```python
from build123d import *

# Parameters (mm, degrees)
BASE_FLANGE1_DEPTH = 156
SKETCH6_R          = 13
CUT_EXTRUDE1_DEPTH = 312.184832535
SKETCH7_R          = 21.05
SKETCH7_R_2        = 2.5
CUT_EXTRUDE2_DEPTH = 10
SKETCH9_R          = 19.05
SKETCH9_R_2        = 2.5
CUT_EXTRUDE3_DEPTH = 10
SKETCH10_R         = 13
CUT_EXTRUDE4_DEPTH = 10
SKETCH12_R         = 13
CUT_EXTRUDE5_DEPTH = 10
SKETCH14_R         = 3
CUT_EXTRUDE6_DEPTH = 10
SKETCH15_R         = 3
CUT_EXTRUDE7_DEPTH = 10
CUT_EXTRUDE8_DEPTH = 312.184832535
FILLET1_R          = 50
FILLET2_R          = 40
SKETCH16_R         = 3
CUT_EXTRUDE9_DEPTH = 10


# Sheet-metal steps are written as plain solids
with BuildPart() as part:
    # Sketch1 → Base-Flange1 (new body)
    with BuildSketch(Plane.XY):
        with BuildLine():
            Line((-77.380352645, 230), (-77.380352645, 3))
            ThreePointArc((-77.380352645, 3), (-76.501672988, 0.878679656), (-74.380352645, 0))
            Line((-74.380352645, 0), (53.619647355, 0))
            ThreePointArc((53.619647355, 0), (55.740967699, 0.878679656), (56.619647355, 3))
            Line((56.619647355, 3), (56.619647355, 230))
            Line((56.619647355, 230), (59.619647355, 230))
            Line((59.619647355, 230), (59.619647355, 3))
            ThreePointArc((59.619647355, 3), (57.862288042, -1.242640687), (53.619647355, -3))
            Line((53.619647355, -3), (-74.380352645, -3))
            ThreePointArc((-74.380352645, -3), (-78.622993332, -1.242640687), (-80.380352645, 3))
            Line((-80.380352645, 3), (-80.380352645, 230))
            Line((-80.380352645, 230), (-77.380352645, 230))
        make_face()
    extrude(amount=BASE_FLANGE1_DEPTH)

    # Sketch6 → Cut-Extrude1 (cut, through all)
    with BuildSketch(Plane(origin=(59.619647355, 0, 0), x_dir=(0, 0, -1), z_dir=(1, 0, 0))):
        with Locations((-78, 197)):
            Circle(SKETCH6_R)
    extrude(amount=-CUT_EXTRUDE1_DEPTH, mode=Mode.SUBTRACT)

    # Sketch7 → Cut-Extrude2 (cut)
    with BuildSketch(Plane.ZY.offset(80.380352645)):
        with Locations(Location((114, 100, 0), (0, 0, 270))):
            Circle(SKETCH7_R)
        with Locations(Location((90.43, 123.57, 0), (0, 0, 270))):
            Circle(SKETCH7_R_2)
        with Locations(Location((137.57, 123.57, 0), (0, 0, 270))):
            Circle(SKETCH7_R_2)
        with Locations(Location((137.57, 76.43, 0), (0, 0, 270))):
            Circle(SKETCH7_R_2)
        with Locations(Location((90.43, 76.43, 0), (0, 0, 270))):
            Circle(SKETCH7_R_2)
    extrude(amount=-CUT_EXTRUDE2_DEPTH, mode=Mode.SUBTRACT)

    # Sketch9 → Cut-Extrude3 (cut)
    with BuildSketch(Plane(origin=(59.619647355, 0, 0), x_dir=(0, 0, -1), z_dir=(1, 0, 0))):
        with Locations((-114, 40)):
            Circle(SKETCH9_R)
        with Locations((-90.43, 63.57)):
            Circle(SKETCH9_R_2)
        with Locations((-137.57, 63.57)):
            Circle(SKETCH9_R_2)
        with Locations((-137.57, 16.43)):
            Circle(SKETCH9_R_2)
        with Locations((-90.43, 16.43)):
            Circle(SKETCH9_R_2)
    extrude(amount=-CUT_EXTRUDE3_DEPTH, mode=Mode.SUBTRACT)

    # Sketch10 → Cut-Extrude4 (cut)
    with BuildSketch(Plane(origin=(0, 0, 0), x_dir=(1, 0, 0), z_dir=(0, 1, 0))):
        with Locations(Location((-10.380352645, -78, 0), (0, 0, 270))):
            Circle(SKETCH10_R)
    extrude(amount=-CUT_EXTRUDE4_DEPTH, mode=Mode.SUBTRACT)

    # Sketch12 → Cut-Extrude5 (cut)
    with BuildSketch(Plane.XZ.offset(3)):
        with Locations(Location((5.789398738, 44.000000006, 0), (0, 0, 270))):
            Circle(SKETCH12_R)
    extrude(amount=-CUT_EXTRUDE5_DEPTH, mode=Mode.SUBTRACT)

    # Sketch14 → Cut-Extrude6 (cut)
    with BuildSketch(Plane(origin=(59.619647355, 0, 0), x_dir=(0, 0, -1), z_dir=(1, 0, 0))):
        with Locations((-52, 97)):
            Circle(SKETCH14_R)
        with BuildLine():
            ThreePointArc((-46.82612575, 119.41051149), (-68.263455967, 113.263455967), (-74.41051149, 91.82612575))
            ThreePointArc((-74.41051149, 91.82612575), (-70.812548133, 89.577868719), (-68.564291101, 93.175832076))
            ThreePointArc((-68.564291101, 93.175832076), (-64.02081528, 109.02081528), (-48.175832076, 113.564291101))
            ThreePointArc((-48.175832076, 113.564291101), (-44.577868719, 115.812548133), (-46.82612575, 119.41051149))
        make_face()
        with BuildLine():
            ThreePointArc((-41.427300446, 142.795393045), (-85.234018716, 130.234018716), (-97.795393045, 86.427300446))
            ThreePointArc((-97.795393045, 86.427300446), (-94.197429688, 84.179043415), (-91.949172656, 87.777006772))
            ThreePointArc((-91.949172656, 87.777006772), (-80.991378029, 125.991378029), (-42.777006772, 136.949172656))
            ThreePointArc((-42.777006772, 136.949172656), (-39.179043415, 139.197429688), (-41.427300446, 142.795393045))
        make_face()
    extrude(amount=-CUT_EXTRUDE6_DEPTH, mode=Mode.SUBTRACT)

    # Sketch15 → Cut-Extrude7 (cut)
    with BuildSketch(Plane(origin=(-77.380352645, 0, 0), x_dir=(0, 0, -1), z_dir=(1, 0, 0))):
        with Locations(Location((-43, 160, 0), (0, 0, 90))):
            Circle(SKETCH15_R)
        with BuildLine():
            ThreePointArc((-85.143312097, 179.651749171), (-86.695706867, 144.096063335), (-62.651749171, 117.856687903))
            ThreePointArc((-62.651749171, 117.856687903), (-59.329434049, 119.065911716), (-60.538657862, 122.388226838))
            ThreePointArc((-60.538657862, 122.388226838), (-81.997243763, 145.806164052), (-80.611773162, 177.538657862))
            ThreePointArc((-80.611773162, 177.538657862), (-81.820996975, 180.860972984), (-85.143312097, 179.651749171))
        make_face()
        with BuildLine():
            ThreePointArc((-63.845079102, 169.72022002), (-64.612930278, 152.133536704), (-52.72022002, 139.154920898))
            ThreePointArc((-52.72022002, 139.154920898), (-48.733441874, 140.605989474), (-50.18451045, 144.59276762))
            ThreePointArc((-50.18451045, 144.59276762), (-58.974774553, 154.185657563), (-58.40723238, 167.18451045))
            ThreePointArc((-58.40723238, 167.18451045), (-59.858300956, 171.171288596), (-63.845079102, 169.72022002))
        make_face()
    extrude(amount=-CUT_EXTRUDE7_DEPTH, mode=Mode.SUBTRACT)

    # Sketch13 → Cut-Extrude8 (cut, through all)
    with BuildSketch(Plane(origin=(59.619647355, 0, 0), x_dir=(0, 0, -1), z_dir=(1, 0, 0))):
        Polygon((-100, 230), (-156, 133.005154776), (-156, 230), align=None)
        Polygon((-44, 230), (0, 153.789764467), (0, 230), align=None)
    extrude(amount=-CUT_EXTRUDE8_DEPTH, mode=Mode.SUBTRACT)

    # Fillet1
    # the kernel refuses this fillet: 50 mm, written as the material it takes off along each edge
    with BuildSketch(Plane(origin=(131.788431004, 230, 44), x_dir=(0, -0.8660254037844418, -0.49999999999999445), z_dir=(-1, 0, 0)), Plane(origin=(-5.211568996, 230, 44), x_dir=(0, -0.8660254037844418, -0.49999999999999445), z_dir=(-1, 0, 0))) as fillet1_piece_1:
        with BuildLine():
            CenterArc((FILLET1_R * 0.57735026919, FILLET1_R), FILLET1_R, 210, 60)
            Line((-FILLET1_R * 0.288675134595, FILLET1_R * 0.5), (0, 0))
            Line((0, 0), (FILLET1_R * 0.57735026919, 0))
        make_face()
    extrude(amount=147.337567297, mode=Mode.SUBTRACT)
    with BuildSketch(Plane(origin=(-5.211568996, 230, 100), x_dir=(0, -0.8660254037844418, 0.49999999999999445), z_dir=(-1, 0, 0)), Plane(origin=(131.788431004, 230, 100), x_dir=(0, -0.8660254037844418, 0.49999999999999445), z_dir=(-1, 0, 0))) as fillet1_piece_2:
        with BuildLine():
            CenterArc((FILLET1_R * 0.57735026919, -FILLET1_R), FILLET1_R, 90, 60)
            Line((-FILLET1_R * 0.288675134595, -FILLET1_R * 0.5), (0, 0))
            Line((0, 0), (FILLET1_R * 0.57735026919, 0))
        make_face()
    extrude(amount=147.337567297, mode=Mode.SUBTRACT)

    # Fillet2
    fillet2_edges = [part.edges().sort_by_distance(p)[0] for p in [
        (58.119647355, 153.789764467, 0),
        (58.119647355, 133.005154776, 156),
        (-78.880352645, 133.005154776, 156),
        (-78.880352645, 153.789764467, 0),
    ]]
    fillet(fillet2_edges, radius=FILLET2_R)

    # Sketch16 → Cut-Extrude9 (cut)
    with BuildSketch(Plane.XZ.offset(3)):
        with Locations(Location((-54.380352645, 129, 0), (0, 0, 270))):
            Circle(SKETCH16_R)
        with Locations(Location((-54.380352645, 105, 0), (0, 0, 270))):
            Circle(SKETCH16_R)
        with Locations(Location((-54.380352645, 55.647353532, 0), (0, 0, 270))):
            Circle(SKETCH16_R)
        with Locations(Location((-54.380352645, 31.647353532, 0), (0, 0, 270))):
            Circle(SKETCH16_R)
        with Locations(Location((33.619647355, 129, 0), (0, 0, 270))):
            Circle(SKETCH16_R)
        with Locations(Location((33.619647355, 105, 0), (0, 0, 270))):
            Circle(SKETCH16_R)
        with Locations(Location((33.619647355, 55.647353532, 0), (0, 0, 270))):
            Circle(SKETCH16_R)
        with Locations(Location((33.619647355, 31.647353532, 0), (0, 0, 270))):
            Circle(SKETCH16_R)
    extrude(amount=-CUT_EXTRUDE9_DEPTH, mode=Mode.SUBTRACT)


solid = part.part
```
Can you work these out from the model? Positions are in its coordinate system, mm. A direction names the side the tool comes from. Give positions to 0.01 mm unless a question says otherwise; leave off trailing zeros. Write each loop counter-clockwise with the first axis right and the second up, starting at its lowest first coordinate (ties: lowest second). Pieces come first, ordered by that corner, then holes. Notation, with made-up numbers: (-10.5, 2.25) -> (28.5, 2.25) arc R19 cw to (28.5, 11.25) -> close; hole circle Ø11 at (80.25, 45). An arc over 180 degrees is marked (long way). Write item = value, one per line.
(1) For faces 1 (the face through (58.141, 16.54, 92.928)), 2 (the face through (-78.901, 90.287, 95.325)), 3 (the face through (-78.859, 184.329, 17.632)), which set-ups out of +Z, -Z, +X, -X, +Y, -Y let a thin tool reach every point of the face, with its end or its side?
Worked out:
face_1 = +X
face_2 = -X
face_3 = -Z, +X, -X, +Y
(2) Suppose I cut it at C-C on y = 160. Write out the boundary of the cut face in (x, z), then the cut area to 3 significant figures.
Worked out:
outline = (-80.38, 3.76) -> (-77.38, 3.76) -> (-77.38, 40) -> (-80.38, 40) -> close; (-80.38, 46) -> (-77.38, 46) -> (-77.38, 60) -> (-80.38, 60) -> close; (-80.38, 66) -> (-77.38, 66) -> (-77.38, 84.5) -> (-80.38, 84.5) -> close; (-80.38, 89.5) -> (-77.38, 89.5) -> (-77.38, 140.41) -> (-80.38, 140.41) -> close; (56.62, 3.76) -> (59.62, 3.76) -> (59.62, 140.41) -> (56.62, 140.41) -> close
area = 769 mm^2
(3) Suppose I cut it at D-D on x = 26. Write out the boundary of the cut face in (y, z).
Worked out:
outline = (-3, 0) -> (0, 0) -> (0, 156) -> (-3, 156) -> close
(4) Thinking about a two-plate mould opening in X: for faces 4 (the face through (30.96, -1.52, 30.26)), 5 (the face through (-78.901, 132.498, 154.675)), which applies, released by +X, released by -X, zero draft, split by the parting line, or undercut?
Worked out:
face_4 = undercut
face_5 = zero draft
(5) Suppose I cut it at B-B on y = 50.5. Write out the boundary of the cut face in (x, z).
Worked out:
outline = (-80.38, 0) -> (-77.38, 0) -> (-77.38, 156) -> (-80.38, 156) -> close; (56.62, 0) -> (59.62, 0) -> (59.62, 98.1) -> (56.62, 98.1) -> close; (56.62, 129.9) -> (59.62, 129.9) -> (59.62, 156) -> (56.62, 156) -> close
(6) I'm going to push flat-ended pins straight in: P1, Ø4.5, axis at y = 63.57, z = 90.43, coming from the +X side; P2, Ø7, axis at x = 33.62, z = 31.65, coming from the +Y side. Where does each tip first touch, or does it pass through?
Worked out:
P1 = -77.38
P2 = 0
(7) Suppose I cut it at A-A on z = 118. Write out the boundary of the cut face in (x, y), then the cut area to 3 significant figures.
Worked out:
outline = (-80.38, 3) arc R6 ccw to (-74.38, -3) -> (53.62, -3) arc R6 ccw to (59.62, 3) -> (59.62, 21.37) -> (56.62, 21.37) -> (56.62, 3) arc R3 cw to (53.62, 0) -> (-74.38, 0) arc R3 cw to (-77.38, 3) -> (-77.38, 79.33) -> (-80.38, 79.33) -> close; (-80.38, 120.67) -> (-77.38, 120.67) -> (-77.38, 198.82) -> (-80.38, 198.82) -> close; (56.62, 58.63) -> (59.62, 58.63) -> (59.62, 198.82) -> (56.62, 198.82) -> close
area = 1,370 mm^2
(8) I need wall thicknesses on probe 1 along X at (y, z) = (35, 12); probe 2 along X at (y, z) = (-1, 129); probe 3 along Y at (x, z) = (58, 78). Which ranges of each line are inside material? Lowest first, please. Write a range as from..to.
Worked out:
probe_1 = -80.38..-77.38, 56.62..59.62
probe_2 = -78.85..-57.38, -51.38..30.62, 36.62..58.09
probe_3 = -1.1..128.7, 136.15..184, 210..229.53
